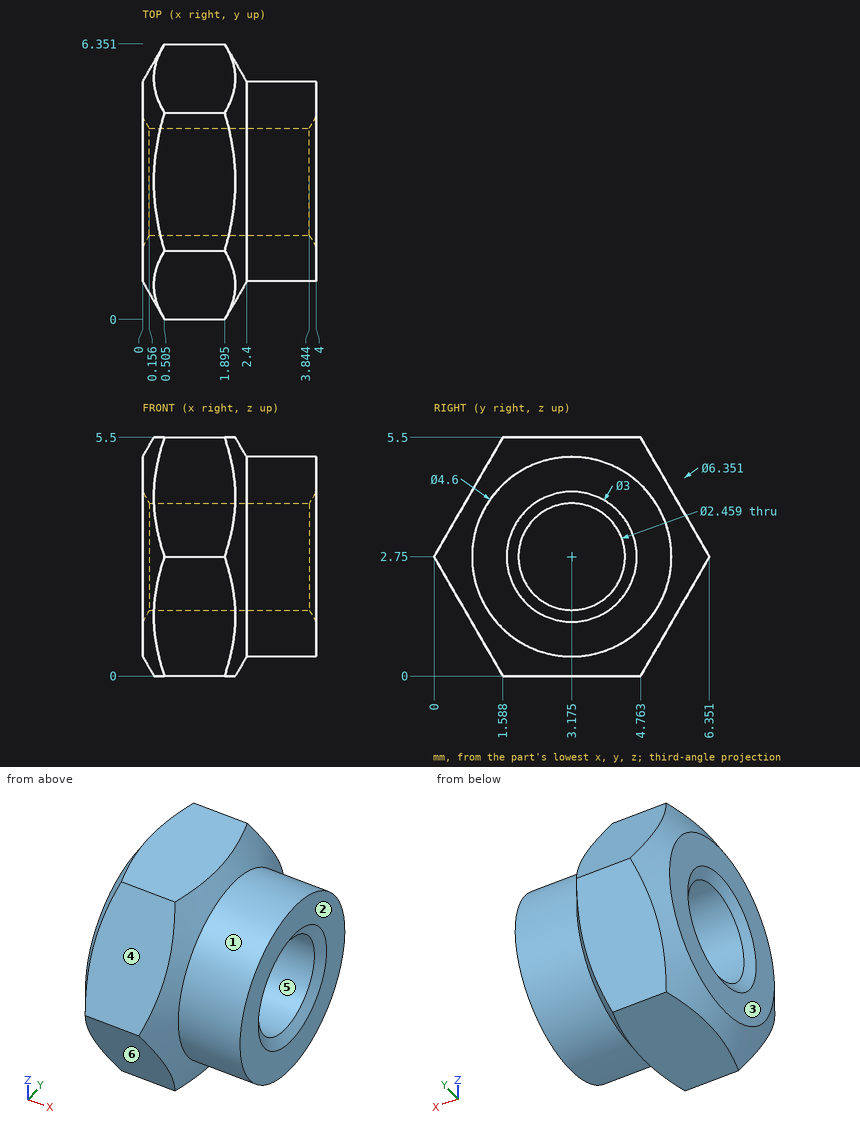
Study the drawing (mm; zero at the part's minimum x, y, z) and answer. A direction names the side the tool comes from. Round coordinates to 2 decimals unless told otherwise and drop trailing zeros.
Q1. For a pull along Z with two mould halves and no side action, classify the marked faces 3, 4, 5 and 6 as released by +Z, released by -Z, zero draft, split by the parting line, or undercut.
Q2. Given pin 1 Ø1 at (x, y) = (1.5, 5.5) entering from +Z; pin 2 Ø1 at (x, y) = (3, 5) entering from +Z, each flat-ended and moving along its own axis, determine where each tip first touches the part or whether it passes through.
Q3. Find the intervals of material crossed by line 1 (Y direction, x = 3.15, z = 2.75) (1 decimal); line 2 (Z direction, x = 1.3, y = 3.25); line 3 (Y direction, x = 2.55, z = 2.85), in increasing order.
Q4. Which of the six approach directions +Z, -Z, +X, -X, +Y, -Y give full straight-line access (tool end or side, diameter ignored) to the marked faces 1 and 2?
Completed:
1. face 3: zero draft
1. face 4: released by +Z
1. face 5: undercut
1. face 6: released by -Z
2. pin 1: stops at z = 5.09
2. pin 2: stops at z = 4.63
3. line 1: y = 0.9 to 1.9, 4.4 to 5.5
3. line 2: z = 0 to 1.52, 3.98 to 5.5
3. line 3: y = 0.88 to 1.95, 4.4 to 5.47
4. face 1: +X
4. face 2: +Z, -Z, +X, +Y, -Y
